from build123d import *

# Parameters (mm, degrees)
SKETCH2_W           = 203.2
SKETCH2_H           = 88.9
SKETCH2_R           = 3.5
SKETCH2_R_2         = 10
BOSS_EXTRUDE1_DEPTH = 1.27
SKETCH3_R           = 2.5
CUT_EXTRUDE1_DEPTH  = 111.92706658


with BuildPart() as part:
    # Sketch2 → Boss-Extrude1 (new, symmetric)
    with BuildSketch(Plane.XY):
        Rectangle(SKETCH2_W, SKETCH2_H)
        with Locations((-76.2, 23.57)):
            Circle(SKETCH2_R, mode=Mode.SUBTRACT)
        with Locations((-29.06, 23.57)):
            Circle(SKETCH2_R, mode=Mode.SUBTRACT)
        with Locations((-29.06, -23.57)):
            Circle(SKETCH2_R, mode=Mode.SUBTRACT)
        with Locations((-76.2, -23.57)):
            Circle(SKETCH2_R, mode=Mode.SUBTRACT)
        with Locations((29.06, -23.57)):
            Circle(SKETCH2_R, mode=Mode.SUBTRACT)
        with Locations((76.2, -23.57)):
            Circle(SKETCH2_R, mode=Mode.SUBTRACT)
        with Locations((76.2, 23.57)):
            Circle(SKETCH2_R, mode=Mode.SUBTRACT)
        with Locations((29.06, 23.57)):
            Circle(SKETCH2_R, mode=Mode.SUBTRACT)
        Circle(SKETCH2_R_2, mode=Mode.SUBTRACT)
    extrude(amount=BOSS_EXTRUDE1_DEPTH, both=True)

    # Sketch3 → Cut-Extrude1 (cut, through all)
    with BuildSketch(Plane.XY.offset(1.27)):
        with Locations((-92.075, 34.925)):
            Circle(SKETCH3_R)
        with Locations((-92.075, -34.925)):
            Circle(SKETCH3_R)
        with Locations((92.075, -34.925)):
            Circle(SKETCH3_R)
        with Locations((92.075, 34.925)):
            Circle(SKETCH3_R)
    extrude(amount=-CUT_EXTRUDE1_DEPTH, mode=Mode.SUBTRACT)


solid = part.part
Design review of the part built by this model. Coordinates are the model's own, in mm. Coordinates: 2 decimals unless noted, no trailing zeros. Order: outer loops, then holes, each group sorted by start corner. A loop starts at its lowest first (then second) coordinate and runs counter-clockwise, first axis right, second up.
Item 1: For line 1 (Y direction, x = 76.2, z = 0.1); line 2 (Y direction, x = -92, z = 0.35); line 3 (Y direction, x = 0, z = 0.45), list the stretches that pass through material, from the lowest coordinate up.
Item 2: Take a section at A-A, the plane x = 76.2. Write out the cut boundary in (y, z).
Item 3: For pin 1 Ø3 at (x, y) = (-92.075, -34.925) entering from +Z, flat-tipped, find the tip position at first contact; note if it passes through.
Item 4: Take a section at C-C, the plane z = 0.45. Count the separate pieces of the cut face and the enclosed holes in it, then the cut area to 3 significant figures.
Item 5: Take a section at B-B, the plane y = 0. Write out the cut boundary in (x, z), then the cut area to 3 significant figures.
The answers:
1. line 1: y = -44.45 to -27.07, -20.07 to 20.07, 27.07 to 44.45
1. line 2: y = -44.45 to -37.42, -32.43 to 32.43, 37.42 to 44.45
1. line 3: y = -44.45 to -10, 10 to 44.45
2. outline: (-44.45, -1.27) - (-27.07, -1.27) - (-27.07, 1.27) - (-44.45, 1.27) - close; (-20.07, -1.27) - (20.07, -1.27) - (20.07, 1.27) - (-20.07, 1.27) - close; (27.07, -1.27) - (44.45, -1.27) - (44.45, 1.27) - (27.07, 1.27) - close
3. pin 1: passes through
4. separate pieces: 1
4. enclosed holes: 13
4. area: 17,400 mm2
5. outline: (-101.6, -1.27) - (-10, -1.27) - (-10, 1.27) - (-101.6, 1.27) - close; (10, -1.27) - (101.6, -1.27) - (101.6, 1.27) - (10, 1.27) - close
5. area: 465 mm2
